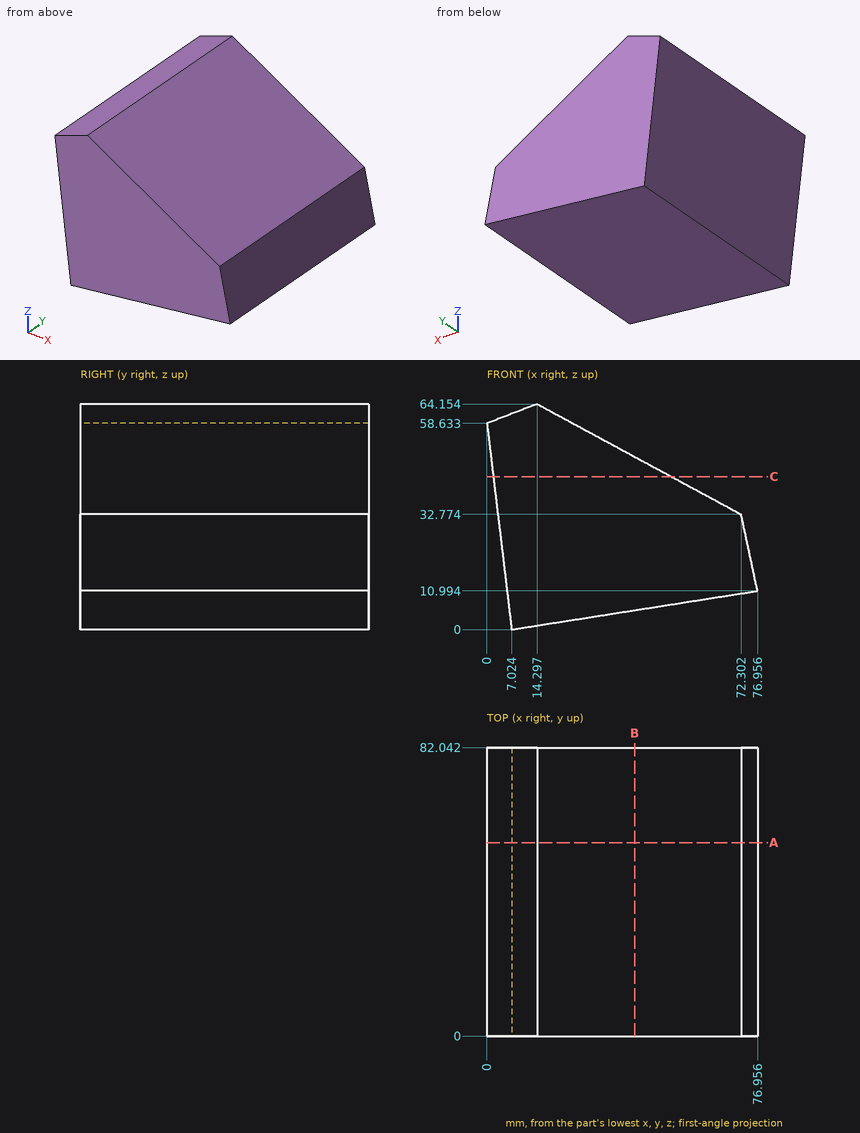
Can you work these out from the drawing? Everything is in mm from the part's minimum corner. Coordinates: 2 decimals unless noted, no trailing zeros. Loops run counter-clockwise (first coordinate to the right, second up) from the corner with the lowest first, then second, coordinate; pieces in that order, holes last.
1. Imagine slicing it at C-C, the plane z = 43.5. Please give me the cut outline in (x, y).
2. For P1, Ø2, axis at x = 68, y = 55, coming from the -Z side; P2, Ø8, axis at x = 38.5, y = 21.5, coming from the +Z side (1 decimal); P3, Ø6, axis at x = 68.5, y = 16.5, coming from the +Z side (1 decimal), each with a flat end and sliding along its axis, tell me the tip position at first contact or that it passes through.
3. Imagine slicing it at B-B, the plane x = 42. Please give me the cut outline in (y, z).
4. Imagine slicing it at A-A, the plane y = 55. Please give me the cut outline in (x, z) (1 decimal), and give its area (3 significant figures).
5. I need wall thicknesses on L1, parallel to Z at x = 42.5, y = 51 (1 decimal); L2, parallel to X at y = 22, z = 27 (1 decimal); L3, parallel to X at y = 17, z = 12 (1 decimal). Which ranges of each line are inside material? Lowest first, please.
Taken from the geometry:
1. outline: (1.81, 0) - (52.48, 0) - (52.48, 82.04) - (1.81, 82.04) - close
2. P1: stops at z = 9.43
2. P2: stops at z = 53.2
2. P3: stops at z = 36.5
3. outline: (0, 5.5) - (82.04, 5.5) - (82.04, 49.17) - (0, 49.17) - close
4. outline: (0, 58.6) - (7, 0) - (77, 11) - (72.3, 32.8) - (14.3, 64.2) - close
4. area: 3,200 mm2
5. L1: z = 5.6 to 48.9
5. L2: x = 3.8 to 73.5
5. L3: x = 5.6 to 76.7
